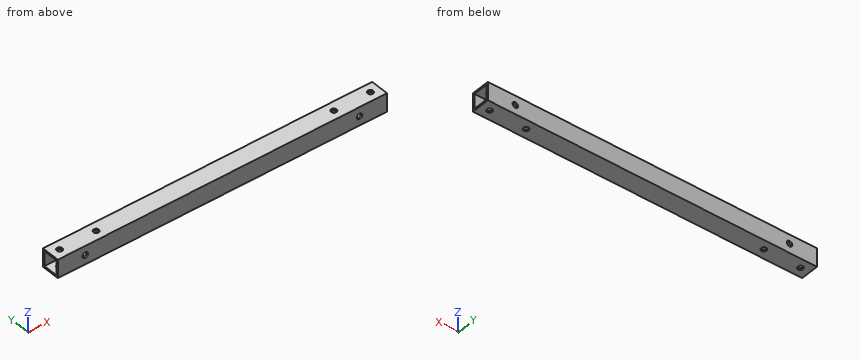
Autodesk Inventor part; units mm, degrees
ref_plane "YZ Plane" through (0, 0, 0) normal (1, 0, 0) x (0, 1, 0)
ref_plane "XZ Plane" through (0, 0, 0) normal (0, 1, 0) x (-1, 0, 0)
ref_plane "XY Plane" through (0, 0, 0) normal (0, 0, 1) x (1, 0, 0)
sketch "スケッチ1" plane through (0, 0, 0) normal (1, 0, 0) x (0, 1, 0)
  line L0 (5, 5) -> (-5, 5)
  line L1 (-5, 5) -> (-5, -5)
  line L2 (-5, -5) -> (5, -5)
  line L3 (5, -5) -> (5, 5)
  line L4 (4, 4) -> (-4, 4)
  line L5 (-4, 4) -> (-4, -4)
  line L6 (-4, -4) -> (4, -4)
  line L7 (4, -4) -> (4, 4)
  point P0 (0, 0)
  dimension "d0" = 1
  dimension "d1" = 1
  dimension "d2" = 1
  dimension "d3" = 1
  dimension "d4" = 10
  dimension "d5" = 10
  dimension "d6" = 5
  dimension "d7" = 5
extrude "押し出し1" add sketch "スケッチ1" along normal blind 180
sketch "スケッチ2" plane through (0, -5, 5) normal (0, 0, 1) x (1, 0, 0)
  circle A0 centre (5, 5) radius 1.5
  circle A1 centre (175, 5) radius 1.5
  line L0 (180, 10) -> (180, 0)
  line L1 (0, 0) -> (180, 0)
  line L2 (0, 10) -> (0, 0)
  line L3 (0, 10) -> (180, 10)
  point P0 (0, 5)
  dimension "d10" = 5
  dimension "d11" = 3
  dimension "d12" = 5
  dimension "d13" = 3
  dimension "d14" = 5
  dimension "d15" = 5
extrude "押し出し2" cut sketch "スケッチ2" against normal blind 200 contours A0 | A1
sketch "スケッチ3" plane through (0, -5, -5) normal (0, -1, 0) x (1, 0, 0)
  circle A0 centre (15, 5) radius 1.5
  line L0 (0, 10) -> (0, 0)
  line L1 (0, 0) -> (180, 0)
  circle A1 centre (165, 5) radius 1.5
  line L2 (180, 10) -> (180, 0)
  line L3 (0, 10) -> (180, 10)
  point P0 (0, 5)
  dimension "d18" = 15
  dimension "d19" = 3
  dimension "d20" = 5
  dimension "d21" = 3
  dimension "d22" = 15
  dimension "d23" = 5
extrude "押し出し3" cut sketch "スケッチ3" against normal blind 200 contours A0 | A1
sketch "スケッチ4" plane through (0, -5, 5) normal (0, 0, 1) x (1, 0, 0)
  circle A0 centre (25, 5) radius 1.5
  circle A1 centre (155, 5) radius 1.5
  line L0 (0, 10) -> (0, 0)
  line L1 (0, 0) -> (180, 0)
  line L2 (180, 10) -> (180, 0)
  point P0 (0, 5)
  dimension "d26" = 25
  dimension "d27" = 3
  dimension "d28" = 5
  dimension "d29" = 5
  dimension "d30" = 25
  dimension "d31" = 3
extrude "押し出し4" cut sketch "スケッチ4" against normal blind 200
properties part number "モーターパーツ３" material "アルミニウム 6061"
Check sheet for the modelled part. Datum: model origin and axes. Units: mm. Round coordinates to 2 decimals unless told otherwise and drop trailing zeros. Order: outer loops, then holes, each group sorted by start corner. A loop starts at its lowest first (then second) coordinate and runs counter-clockwise, first axis right, second up.
(1) Cross-section at D-D, the plane y = 0. State how many separate pieces and enclosed holes the cut face has, and give its area (3 significant figures).
(2) Cross-section at A-A, the plane x = 67.5. Enter the section's corners in (y, z), and give its area (3 significant figures).
(3) Cross-section at B-B, the plane z = 0. Enter the section's corners in (x, y), and give its area (3 significant figures).
(4) Cross-section at C-C, the plane x = 25. Enter the section's corners in (y, z), and give its area (3 significant figures).
(5) Scan lines: probe 1 along Z at (x, y) = (47, -0.5); probe 2 along Y at (x, z) = (5, -4.7). Record each from-to range of solid material in increasing order.
Check sheet entries:
1. separate pieces: 10
1. enclosed holes: 0
1. area: 336 mm2
2. outline: (-5, -5) - (5, -5) - (5, 5) - (-5, 5) - close; hole (-4, -4) - (4, -4) - (4, 4) - (-4, 4) - close
2. area: 36.0 mm2
3. outline: (0, -5) - (13.5, -5) - (13.5, -4) - (0, -4) - close; (0, 4) - (13.5, 4) - (13.5, 5) - (0, 5) - close; (16.5, -5) - (163.5, -5) - (163.5, -4) - (16.5, -4) - close; (16.5, 4) - (163.5, 4) - (163.5, 5) - (16.5, 5) - close; (166.5, -5) - (180, -5) - (180, -4) - (166.5, -4) - close; (166.5, 4) - (180, 4) - (180, 5) - (166.5, 5) - close
3. area: 348 mm2
4. outline: (-5, -5) - (-1.5, -5) - (-1.5, -4) - (-4, -4) - (-4, 4) - (-1.5, 4) - (-1.5, 5) - (-5, 5) - close; (1.5, -5) - (5, -5) - (5, 5) - (1.5, 5) - (1.5, 4) - (4, 4) - (4, -4) - (1.5, -4) - close
4. area: 30.0 mm2
5. probe 1: z = -5 to -4, 4 to 5
5. probe 2: y = -5 to -1.5, 1.5 to 5
